from build123d import *

# Parameters (mm, degrees)
SKETCH1_R           = 10
SKETCH1_R_2         = 7.5
BOSS_EXTRUDE1_DEPTH = 98
SKETCH2_R           = 7.5
BOSS_EXTRUDE2_DEPTH = 5
SKETCH3_R           = 3.5
CUT_EXTRUDE1_DEPTH  = 5
SKETCH4_R           = 7.5
BOSS_EXTRUDE4_DEPTH = 3
SKETCH5_R           = 6.688248189
CUT_EXTRUDE2_DEPTH  = 5


with BuildPart() as part:
    # Sketch1 → Boss-Extrude1 (new body)
    with BuildSketch(Plane.XY):
        Circle(SKETCH1_R)
        Circle(SKETCH1_R_2, mode=Mode.SUBTRACT)
    extrude(amount=BOSS_EXTRUDE1_DEPTH)

    # Sketch2 → Boss-Extrude2 (add)
    with BuildSketch(Plane.XY.offset(98)):
        Circle(SKETCH2_R)
    extrude(amount=-BOSS_EXTRUDE2_DEPTH)

    # Sketch3 → Cut-Extrude1 (cut)
    with BuildSketch(Plane.XY.offset(98)):
        Circle(SKETCH3_R)
    extrude(amount=-CUT_EXTRUDE1_DEPTH, mode=Mode.SUBTRACT)

    # Sketch4 → Boss-Extrude4 (add)
    with BuildSketch(Plane(origin=(0, 0, 0), x_dir=(-1, 0, 0), z_dir=(0, 0, -1))):
        Circle(SKETCH4_R)
    extrude(amount=-BOSS_EXTRUDE4_DEPTH)

    # Sketch5 → Cut-Extrude2 (cut)
    with BuildSketch(Plane(origin=(0, 0, 0), x_dir=(-1, 0, 0), z_dir=(0, 0, -1))):
        Circle(SKETCH5_R)
    extrude(amount=-CUT_EXTRUDE2_DEPTH, mode=Mode.SUBTRACT)


solid = part.part
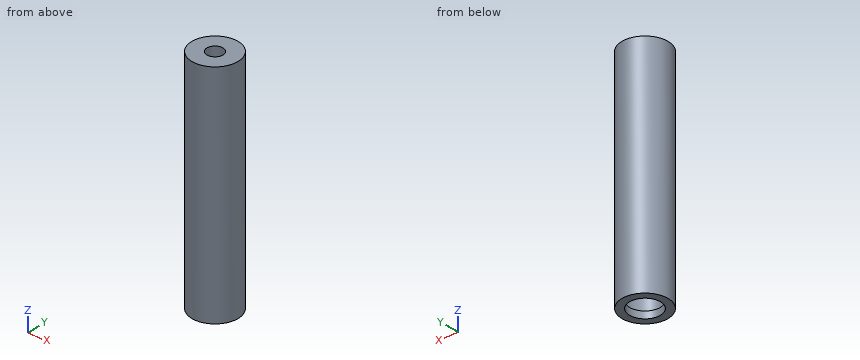
The model under review builds one solid part; all positions refer to its coordinate system, in mm. Round coordinates to 2 decimals unless told otherwise and drop trailing zeros. Order: outer loops, then holes, each group sorted by start corner. A loop starts at its lowest first (then second) coordinate and runs counter-clockwise, first axis right, second up. Notation, with made-up numbers: (-26.5, 10) - (20.5, 10) arc R15 ccw to (20.5, 24) - close; hole circle Ø2 at (-39.75, -22). An arc over 180 degrees is marked (long way). Use one line per item in the form item = value.
Q1. Add section A-A on y = 0. Give the boundary of the cut face in (x, z), then the cut area to 3 significant figures.
Response values:
outline = (-10, 0) - (-6.69, 0) - (-6.69, 3) - (-7.5, 3) - (-7.5, 93) - (-3.5, 93) - (-3.5, 98) - (-10, 98) - close; (3.5, 93) - (7.5, 93) - (7.5, 3) - (6.69, 3) - (6.69, 0) - (10, 0) - (10, 98) - (3.5, 98) - close
area = 535 mm^2
Q2. Clearance check with flat-ended pins moving along their axes: P1, Ø6, axis at y = 4.5, z = 42, coming from the -X side; P2, Ø4, axis at x = 3, z = 58, coming from the +Y side; P3, Ø6, axis at y = -7.5, z = 60.5, coming from the +X side. State where each tip first meets the part, or that it passes through.
Response values:
P1 = -9.89
P2 = 9.95
P3 = 8.93
Q3. Add section D-D on y = 8.5. Give the boundary of the cut face in (x, z).
Response values:
outline = (-5.27, 0) - (5.27, 0) - (5.27, 98) - (-5.27, 98) - close
Q4. Add section C-C on z = 73. Give the boundary of the cut face in (x, y), then the cut area to 3 significant figures.
Response values:
outline = circle Ø20 at (0, 0); hole circle Ø15 at (0, 0)
area = 137 mm^2
Q5. Add section B-B on x = -1.25. Give the boundary of the cut face in (y, z), then the cut area to 3 significant figures.
Response values:
outline = (-9.92, 0) - (-6.57, 0) - (-6.57, 3) - (-7.4, 3) - (-7.4, 93) - (-3.27, 93) - (-3.27, 98) - (-9.92, 98) - close; (3.27, 93) - (7.4, 93) - (7.4, 3) - (6.57, 3) - (6.57, 0) - (9.92, 0) - (9.92, 98) - (3.27, 98) - close
area = 541 mm^2
Q6. To check wall thickness, follow line 1 (Y direction, x = 0, z = 97); line 2 (Z direction, x = -0.25, y = 7.25); line 3 (Z direction, x = 1.5, y = -5.5). State the ranges of each line that lie inside material, in increasing order.
Response values:
line_1 = -10 to -3.5, 3.5 to 10
line_2 = 0 to 3, 93 to 98
line_3 = 93 to 98
